Source: CAD feature listing. Evaluate the final solid. Frame: model axes, mm. Give positions to 0.01 mm unless a question says otherwise; leave off trailing zeros. Loops run counter-clockwise (first coordinate to the right, second up) from the corner with the lowest first, then second, coordinate; pieces in that order, holes last. Notation, with made-up numbers: M -21,89.25 L -14,89.25 A32 ccw -14,123.25 Z; hole C 20.25,71 d2. An arc over 180 degrees is marked long. Answer in a Markdown table with one row per item.
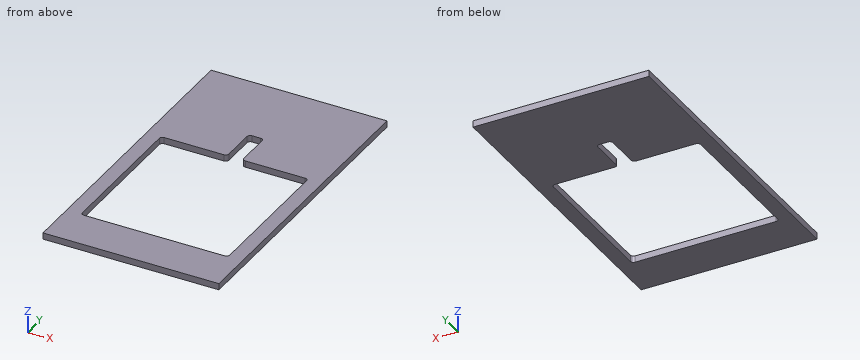
```python
from build123d import *

# Parameters (mm, degrees)
F0_W     = 178.59375
F0_H     = 312.7375
F1_DEPTH = 6.5532
F3_DEPTH = 25.4


with BuildPart() as f1:
    # F0 (on Top) → F1 (new body)
    with BuildSketch(Plane.XY):
        with Locations((89.296875, 156.36875)):
            Rectangle(F0_W, F0_H)
    extrude(amount=F1_DEPTH)

    # F2 (on face) → F3 (cut)
    with BuildSketch(Plane.XY.offset(6.5532)):
        with BuildLine():
            Line((78.501875, 192.9511), (17.7292, 192.9511))
            ThreePointArc((17.7292, 192.9511), (15.484136, 192.021164), (14.5542, 189.7761))
            Line((14.5542, 189.7761), (14.5542, 46.736))
            ThreePointArc((14.5542, 46.736), (15.484136, 44.490936), (17.7292, 43.561))
            Line((17.7292, 43.561), (160.86455, 43.561))
            ThreePointArc((160.86455, 43.561), (163.109614, 44.490936), (164.03955, 46.736))
            Line((164.03955, 46.736), (164.03955, 189.7761))
            ThreePointArc((164.03955, 189.7761), (163.109614, 192.021164), (160.86455, 192.9511))
            Line((160.86455, 192.9511), (100.091875, 192.9511))
            ThreePointArc((100.091875, 192.9511), (97.846811, 193.881036), (96.916875, 196.1261))
            Line((96.916875, 196.1261), (96.916875, 229.9081))
            ThreePointArc((96.916875, 229.9081), (95.986939, 232.153164), (93.741875, 233.0831))
            Line((93.741875, 233.0831), (84.851875, 233.0831))
            ThreePointArc((84.851875, 233.0831), (82.606811, 232.153164), (81.676875, 229.9081))
            Line((81.676875, 229.9081), (81.676875, 196.1261))
            ThreePointArc((81.676875, 196.1261), (80.746939, 193.881036), (78.501875, 192.9511))
        make_face()
    extrude(amount=-F3_DEPTH, mode=Mode.SUBTRACT)


solid = f1.part
```
1) Section C-C, the plane x = 123.5. Return loops of the section in (y, z), then the cut area to 3 significant figures.
Reply:
| item | result |
|---|---|
| outline | M 0,0 L 43.56,0 L 43.56,6.55 L 0,6.55 Z; M 192.95,0 L 312.74,0 L 312.74,6.55 L 192.95,6.55 Z |
| area | 1,070 mm² |
2) Section A-A, the plane y = 168.5. Return loops of the section in (x, z), then the cut area to 3 significant figures.
Reply:
| item | result |
|---|---|
| outline | M 0,0 L 14.55,0 L 14.55,6.55 L 0,6.55 Z; M 164.04,0 L 178.59,0 L 178.59,6.55 L 164.04,6.55 Z |
| area | 191 mm² |
3) Material intervals for L1, parallel to Y at x = 129, z = 4; L2, parallel to X at y = 102, z = 3.75; L3, parallel to Y at x = 86.5, z = 3, sorted ascending.
Reply:
| item | result |
|---|---|
| L1 | y = 0 to 43.56, 192.95 to 312.74 |
| L2 | x = 0 to 14.55, 164.04 to 178.59 |
| L3 | y = 0 to 43.56, 233.08 to 312.74 |
